Here's how the part is built. I have some questions about the finished solid (model axes, mm). Coordinates: 2 decimals unless noted, no trailing zeros. Write each loop counter-clockwise with the first axis right and the second up, starting at its lowest first coordinate (ties: lowest second). Pieces come first, ordered by that corner, then holes. Notation, with made-up numbers: M 69,47 L 94,47 A22 cw 94,79 Z; hole C -23,30 d7. An arc over 180 degrees is marked long. Write each question's results on one line, items separated by ' | '. Start each with the question number.
Autodesk Inventor part; units mm, degrees
ref_plane "YZ Plane" through (0, 0, 0) normal (1, 0, 0) x (0, 1, 0)
ref_plane "XZ Plane" through (0, 0, 0) normal (0, 1, 0) x (-1, 0, 0)
ref_plane "XY Plane" through (0, 0, 0) normal (0, 0, 1) x (1, 0, 0)
sketch "Sketch1" plane through (0, 0, 0) normal (0, 1, 0) x (-1, 0, 0)
  line L0 (95, -95) -> (-95, -95)
  line L1 (-95, -95) -> (-95, 95)
  line L2 (-95, 95) -> (95, 95)
  line L3 (95, 95) -> (95, -95)
  line L4 (95, -95) -> (-95, 95) construction
  line L5 (-95, -95) -> (95, 95) construction
  point P0 (0, 0)
  point P1 (0, 0)
  point P2 (0, 0)
  dimension "d25" = 190
extrude "Extrusion1" add sketch "Sketch1" along normal blind 2.3813
sketch "Sketch2" plane through (0, 2.3813, 0) normal (0, 1, 0) x (1, 0, 0)
  line L0 (-95, -95) -> (95, -95)
  point P0 (0, 0)
  point P1 (0, -85)
  dimension "d26" = 10
hole "Hole1" at (0, 2.3813, 85) direction (0, -1, 0) diameter 5.5 end through all
pattern_circular "Circular Pattern1" count 4 over 360 about axis through (0, -10, 0) along (0, 1, 0) of "Hole1"
sketch "Sketch3" plane through (0, 0, 0) normal (0, -1, 0) x (1, 0, 0)
  circle A0 centre (-85, 0) radius 2.75
  circle A1 centre (0, -85) radius 2.75
  circle A2 centre (85, 0) radius 2.75
  circle A3 centre (0, 85) radius 2.75
  line L0 (-95, -95) -> (95, -95)
  line L1 (95, -95) -> (95, 95)
  line L2 (95, 95) -> (-95, 95)
  line L3 (-95, 95) -> (-95, -95)
  line L4 (0, 106.066) -> (106.066, 0)
  line L5 (106.066, 0) -> (0, -106.066)
  line L6 (0, -106.066) -> (-106.066, 0)
  line L7 (-106.066, 0) -> (0, 106.066)
  line L8 (-106.066, 0) -> (106.066, 0) construction
  line L9 (0, -106.066) -> (0, 106.066) construction
  point P0 (0, 0)
  point P1 (0, 0)
  point P2 (0, 0)
  dimension "d27" = 150
  dimension "d28" = 150
extrude "Extrusion2" cut sketch "Sketch3" against normal through all contours L6 L3 L7 L2 L4 L1 L5 L0 | L0 L5 L6 | L6 L7 L3 | L1 L4 L5 | L7 L4 L2 keep common part
sketch "Sketch4" plane through (0, 0, 0) normal (0, -1, 0) x (1, 0, 0)
  line L0 (-11.066, -95) -> (-95, -11.066)
  line L1 (-11.066, -95) -> (11.066, -95)
  line L2 (95, -11.066) -> (11.066, -95)
  line L3 (95, -11.066) -> (95, 11.066)
  line L4 (11.066, 95) -> (95, 11.066)
  line L5 (11.066, 95) -> (-11.066, 95)
  line L6 (-95, 11.066) -> (-11.066, 95)
  line L7 (-95, 11.066) -> (-95, -11.066)
  circle A0 centre (-85, 0) radius 2.75
  circle A1 centre (0, -85) radius 2.75
  circle A2 centre (85, 0) radius 2.75
  circle A3 centre (0, 85) radius 2.75
  line L8 (-36.066, -70) -> (36.066, -70) construction
  line L9 (-29, -70) -> (29, -70) construction
  line L10 (29, -70) -> (29, -21) construction
  line L11 (29, -21) -> (-29, -21) construction
  line L12 (-29, -21) -> (-29, -70) construction
  line L13 (0, -21) -> (0, -70) construction
  point P0 (0, 0)
  point P1 (0, -70)
  dimension "d31" = 25
  dimension "d32" = 58
  dimension "d33" = 49
hole "Hole2" at (-29, 0, -21) at (29, 0, -21) at (29, 0, -70) at (-29, 0, -70) direction (0, 1, 0) diameter 2.6 end through all
equation "\"d7\" = suppourtPanelThickness"
equation "\"d28\" = d27"
equation "\"panelChamfer\" = 75"
equation "\"suppourtPanelThickness\" = 2.38125"
properties part number "piMount" material "Polycarbonate, Clear"
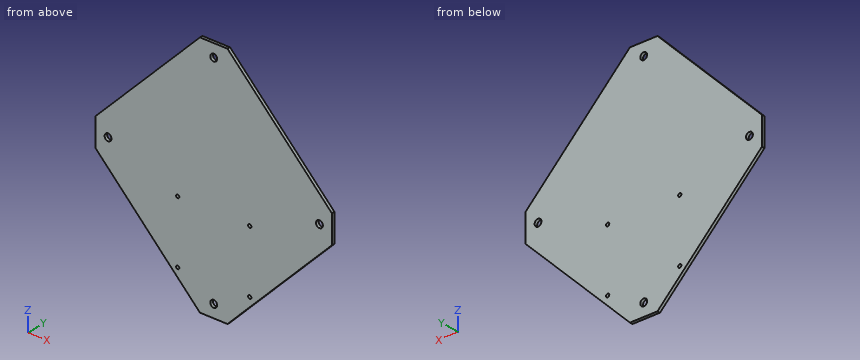
1) I want a section at D-D, the plane x = 85. Write out the boundary of the cut face in (y, z), then the cut area to 3 significant figures.
2) I want a section at C-C, the plane z = 0. Write out the boundary of the cut face in (x, y).
3) Please list where these lines run through material, in increasing order: line 1 (Z direction, x = 0, y = 1.6); line 2 (X direction, y = 0.85, z = -1); line 3 (X direction, y = 1.05, z = -21). Write a range as [from, to].
4) I want a section at A-A, the plane y = 0.45. Give the number of separate pieces and of enclosed holes in the cut face, then the cut area to 3 significant figures.
5) For pin 1 Ø2.5 at (x, z) = (29, -21) entering from +Y; pin 2 Ø1 at (x, y) = (-25, 1) entering from -Z, each with a flat end and sliding along its axis, tell me the tip position at first contact or that it passes through.
6) I want a section at B-B, the plane x = 0. Write out the boundary of the cut face in (y, z), then the cut area to 3 significant figures.
Output:
1) outline: M 0,-21.07 L 2.38,-21.07 L 2.38,-2.75 L 0,-2.75 Z; M 0,2.75 L 2.38,2.75 L 2.38,21.07 L 0,21.07 Z | area: 87.2 mm2
2) outline: M -95,0 L -87.75,0 L -87.75,2.38 L -95,2.38 Z; M -82.25,0 L 82.25,0 L 82.25,2.38 L -82.25,2.38 Z; M 87.75,0 L 95,0 L 95,2.38 L 87.75,2.38 Z
3) line 1: z = [-95, -87.75], [-82.25, 82.25], [87.75, 95] | line 2: x = [-95, -87.56], [-82.44, 82.44], [87.56, 95] | line 3: x = [-85.07, -30.3], [-27.7, 27.7], [30.3, 85.07]
4) separate pieces: 1 | enclosed holes: 8 | area: 21,900 mm2
5) pin 1: passes through | pin 2: stops at z = -81.57
6) outline: M 0,-95 L 2.38,-95 L 2.38,-87.75 L 0,-87.75 Z; M 0,-82.25 L 2.38,-82.25 L 2.38,82.25 L 0,82.25 Z; M 0,87.75 L 2.38,87.75 L 2.38,95 L 0,95 Z | area: 426 mm2
